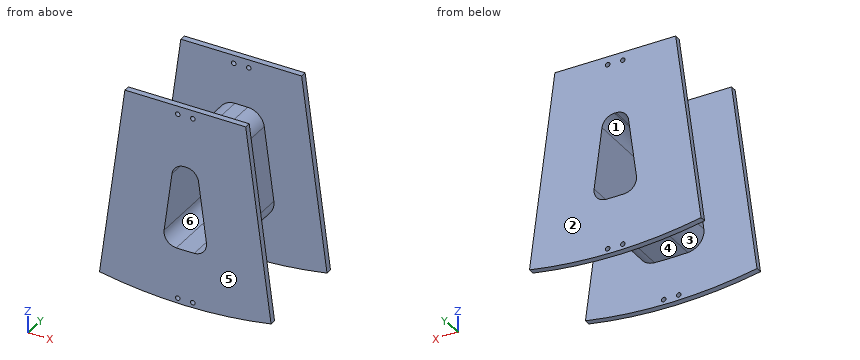
```python
from build123d import *

# Parameters (mm, degrees)
SKETCH1_R           = 1.5
BOSS_EXTRUDE1_DEPTH = 4
BOSS_EXTRUDE2_DEPTH = 60
SCALE1_SCALE        = 0.27
FILLET1_R           = 3
CUT_EXTRUDE1_DEPTH  = 20


with BuildPart() as part:
    # Sketch1 → Boss-Extrude1 (new body)
    with BuildSketch(Plane(origin=(0, 0, 0), x_dir=(1, 0, 0), z_dir=(0, 1, 0))):
        with BuildLine():
            Line((-56.806235592, 60.259400507), (-40, -67.396632609))
            Line((-40, -67.396632609), (40, -67.396632609))
            Line((40, -67.396632609), (56.806235592, 60.259400507))
            ThreePointArc((56.806235592, 60.259400507), (0, 65.5), (-56.806235592, 60.259400507))
        make_face()
        with Locations(Location((-5, 62, 0), (0, 0, 270))):
            Circle(SKETCH1_R, mode=Mode.SUBTRACT)
        with Locations(Location((-5, -62, 0), (0, 0, 270))):
            Circle(SKETCH1_R, mode=Mode.SUBTRACT)
        with Locations(Location((5, -62, 0), (0, 0, 90))):
            Circle(SKETCH1_R, mode=Mode.SUBTRACT)
        with Locations(Location((5, 62, 0), (0, 0, 90))):
            Circle(SKETCH1_R, mode=Mode.SUBTRACT)
    boss_extrude1 = extrude(amount=BOSS_EXTRUDE1_DEPTH)

    # Sketch2 → Boss-Extrude2 (add)
    with BuildSketch(Plane(origin=(0, 4, 0), x_dir=(1, 0, 0), z_dir=(0, 1, 0))):
        with BuildLine():
            Line((13.971014299, -35.267480529), (23.161620791, 34.542106528))
            ThreePointArc((23.161620791, 34.542106528), (0, 35.5), (-23.161620791, 34.542106528))
            Line((-23.161620791, 34.542106528), (-13.971014299, -35.267480529))
            Line((-13.971014299, -35.267480529), (13.971014299, -35.267480529))
        make_face()
    extrude(amount=BOSS_EXTRUDE2_DEPTH)

    # Mirror1: Boss-Extrude1 across plane
    add(boss_extrude1.mirror(Plane.ZX.offset(34)))


with BuildPart() as part_1:
    # Scale1: scaled about (0, 34, -2.563249607)
    add(part.part.scale(SCALE1_SCALE).moved(Location((0, 24.82, -1.871172213))))

    # Fillet1
    fillet1_edges = [part_1.edges().sort_by_distance(p)[0] for p in [
        (3.772173861, 34, 7.65104753),
        (6.253637614, 34, -11.197540976),
        (-6.253637614, 34, -11.197540976),
        (-3.772173861, 34, 7.65104753),
    ]]
    fillet(fillet1_edges, radius=FILLET1_R)

    # Sketch3 → Cut-Extrude1 (cut)
    with BuildSketch(Plane(origin=(0, 43.18, 0), x_dir=(1, 0, 0), z_dir=(0, 1, 0))):
        with BuildLine():
            ThreePointArc((2.373141134, -3.721290728), (1.624743129, -5.12027622), (0.139265082, -5.677604625))
            ThreePointArc((0.139265082, -5.677604625), (0, -5.677507909), (-0.139265082, -5.677604625))
            ThreePointArc((-0.139265082, -5.677604625), (-1.624743129, -5.12027622), (-2.373141134, -3.721290728))
            Line((-2.373141134, -3.721290728), (-3.784051042, 6.995634014))
            ThreePointArc((-3.784051042, 6.995634014), (-3.260936346, 8.754404452), (-1.602122137, 9.538788197))
            ThreePointArc((-1.602122137, 9.538788197), (0, 9.556172213), (1.602122137, 9.538788197))
            ThreePointArc((1.602122137, 9.538788197), (3.260936346, 8.754404452), (3.784051042, 6.995634014))
            Line((3.784051042, 6.995634014), (2.373141134, -3.721290728))
        make_face()
    extrude(amount=-CUT_EXTRUDE1_DEPTH, mode=Mode.SUBTRACT)


solid = part_1.part
```
Part model, mm, in its own coordinate system. Face numbers are marked on the shaded views. A direction names the side the tool comes from. Round coordinates to 2 decimals unless told otherwise and drop trailing zeros. Write each loop counter-clockwise with the first axis right and the second up, starting at its lowest first coordinate (ties: lowest second). Pieces come first, ordered by that corner, then holes. Notation, with made-up numbers: M 72,-4.75 L 88,-4.75 A18 cw 88,29.25 Z; hole C 5,68.25 d5. An arc over 180 degrees is marked long. One line per question, with ' | ' between items.
(1) Saw through at C-C on z = -6.5. Write the cut outline in (x, y).
Answer key:
outline: M -13.81,24.82 L -3.72,24.82 L -3.72,43.18 L -13.81,43.18 L -13.81,42.1 L -5.64,42.1 L -5.64,25.9 L -13.81,25.9 Z; M 3.72,24.82 L 13.81,24.82 L 13.81,25.9 L 5.64,25.9 L 5.64,42.1 L 13.81,42.1 L 13.81,43.18 L 3.72,43.18 Z
(2) Saw through at A-A on y = 38.5. Write the cut outline in (x, z) (3 decimals).
Answer key:
outline: M -5.834,-8.008 A3 ccw -2.977,-11.398 A75.735 ccw 2.977,-11.398 A3 ccw 5.834,-8.008 L 4.116,5.043 A3 ccw 1.141,7.651 L -1.141,7.651 A3 ccw -4.116,5.043 Z; hole M -3.784,-6.996 A2.25 ccw -1.602,-9.539 A73.835 ccw 1.602,-9.539 A2.25 ccw 3.784,-6.996 L 2.373,3.721 A2.25 ccw 0.139,5.678 A100.267 cw -0.139,5.678 A2.25 ccw -2.373,3.721 Z
(3) 3-axis set-ups, long thin cutter, end or side, ignore diameter. For the marked faces 4, 5 and 6: which of +Z, -Z, +X, -X, +Y, -Y reach the whole face in a straight line?
Answer key:
face 4: -Z | face 5: +Z, -Z, +X, -X, -Y | face 6: +Y, -Y
(4) Two-plate mould, pull along X, no slides. Class the marked faces 1, 2 and 3: released by +X, released by -X, zero draft, split by the parting line, or undercut.
Answer key:
face 1: undercut | face 2: zero draft | face 3: released by -X
(5) Saw through at B-B on x = -12. Write the cut outline in (y, z), then the cut area to 3 significant figures.
Answer key:
outline: M 24.82,-18.69 L 25.9,-18.69 L 25.9,7.21 L 24.82,7.21 Z; M 42.1,-18.69 L 43.18,-18.69 L 43.18,7.21 L 42.1,7.21 Z | area: 56.0 mm^2
(6) Probe line 1 along Y through (x, z) = (-3.5, -15); line 2 along Z through (x, y) = (1.35, 25.55); line 3 along X through (y, z) = (35.5, 5.5). List the from-to ranges inside material, lowest first.
Answer key:
line 1: y = 24.82 to 25.9, 42.1 to 43.18 | line 2: z = -19.55 to -19.02, -18.21 to -9.54, 5.33 to 14.46, 15.27 to 16.33 | line 3: x = -4.02 to -1.02, 1.02 to 4.02
(7) Pin check, flat tips, straight feed: pin 1 (2 mm diameter, centred on x = 8.5, y = 34, fed in from -Z); pin 2 (12 mm diameter, centred on x = -11.5, z = 12, fed in from -Y); pin 3 (8 mm diameter, centred on y = 27.5, z = 2.5, fed in from +X); pin 4 (8 mm diameter, centred on y = 40, z = -11, fed in from +X). Stop position of each tip, or through.
Answer key:
pin 1: passes through | pin 2: stops at y = 24.82 | pin 3: stops at x = 13.1 | pin 4: stops at x = 14.85
(8) Saw through at D-D on x = -5. Write the cut outline in (y, z), then the cut area to 3 significant figures.
Answer key:
outline: M 24.82,-19.41 L 25.9,-19.41 L 25.9,-10.5 L 42.1,-10.5 L 42.1,-19.41 L 43.18,-19.41 L 43.18,16.33 L 42.1,16.33 L 42.1,-1.68 L 25.9,-1.68 L 25.9,16.33 L 24.82,16.33 Z | area: 220 mm^2
